```python
from build123d import *

# Parameters (mm, degrees)
F1_DEPTH = 3
F0_W     = 20
F0_H     = 2.5
F0_W_2   = 70
F2_DEPTH = 3
F3_DEPTH = 15
F4_R     = 2


with BuildPart() as f1:
    # F0 (on Top) → F1 (new body)
    with BuildSketch(Plane.XY):
        Polygon((-24.26379, -16.103005), (-24.26379, -22.103005), (-4.26379, -22.103005), (25.73621, -22.103005), (45.73621, -22.103005), (45.73621, -16.103005), align=None)
    extrude(amount=F1_DEPTH)

    # F0 (on Top) → F2 (join)
    with BuildSketch(Plane.XY):
        with Locations((-14.26379, -23.353005)):
            Rectangle(F0_W, F0_H)
        with Locations((35.73621, -23.353005)):
            Rectangle(F0_W, F0_H)
        with Locations((10.73621, -14.853005)):
            Rectangle(F0_W_2, F0_H)
    extrude(amount=F2_DEPTH)

    # F0 (on Top) → F3 (join)
    with BuildSketch(Plane.XY):
        with Locations((10.73621, -14.853005)):
            Rectangle(F0_W_2, F0_H)
        with Locations((-14.26379, -23.353005)):
            Rectangle(F0_W, F0_H)
        with Locations((35.73621, -23.353005)):
            Rectangle(F0_W, F0_H)
    extrude(amount=-F3_DEPTH)

    # F4
    f4_edges = [f1.edges().sort_by_distance(p)[0] for p in [
        (10.73621, -13.603005, 3),
        (-14.26379, -24.603005, 3),
        (35.73621, -24.603005, 3),
    ]]
    fillet(f4_edges, radius=F4_R)


solid = f1.part
```
Geometry: final body of the model. Coordinates: model frame, mm. A direction names the side the tool comes from. Give positions to 0.01 mm unless a question says otherwise; leave off trailing zeros. Loops run counter-clockwise (first coordinate to the right, second up) from the corner with the lowest first, then second, coordinate; pieces in that order, holes last. Notation, with made-up numbers: (28, 81) - (47, 81) arc R15 cw to (47, 96) - close; hole circle Ø11 at (2.25, 52.5). An arc over 180 degrees is marked (long way). Answer as CSV lines item,"result". Start each with the question number.
(1) Reachability of faces 4 (the face through (36, -22.103, -7)), 5 (the face through (10, -19, 3)), 6 (the face through (11, -22.103, 1)) from +Z, -Z, +X, -X, +Y, -Y: full face, straight path, thin tool, end or side. Return the list, or none.
(2) Section query D-D (x = 13). Output: boundary loops of the cut face in (y, z).
(3) Pin query (flat end, axial travel): P1, Ø1.8, axis at x = 5.5, y = -18, coming from the -Z side; P2, Ø7.5, axis at x = 5, z = -6, coming from the -Y side; P3, Ø3.5, axis at x = 14.5, z = 2, coming from the -Y side. Return the tip coordinate at first contact, or that it passes through.
(4) Section query C-C (y = -17.5). Output: boundary loops of the cut face in (x, z), and give its area (3 significant figures).
(5) Mould query, pull axis Y, two halves, no side actions, for faces 1 (the face through (10, -15, -15)), 2 (the face through (10, -13.603, -7)), 3 (the face through (-14, -22.103, -7)). Classes: +Y half, -Y half, draft (parallel to the pull), parting line (faces both ways), or undercut.
(6) Ray query, line 1 along Y through (x, z) = (-19.5, -5.25); line 2 along X through (y, z) = (-24, -2.25); line 3 along Y through (x, z) = (21.5, -13.5). Return the intervals inside material, ascending. Write a range as [from, to].
(7) Section query B-B (x = 40). Output: boundary loops of the cut face in (y, z).
(8) Section query A-A (z = -12.5). Output: boundary loops of the cut face in (x, y).
Worked answers:
1,face 4,"-Z, +X, -X"
1,face 5,"+Z, +X, -X, +Y, -Y"
1,face 6,"+Z, -Z, -Y"
2,outline,"(-22.1, 0) - (-16.1, 0) - (-16.1, -15) - (-13.6, -15) - (-13.6, 1) arc R2 ccw to (-15.6, 3) - (-22.1, 3) - close"
3,P1,"stops at z = 0"
3,P2,"stops at y = -16.1"
3,P3,"stops at y = -22.1"
4,outline,"(-24.26, 0) - (45.74, 0) - (45.74, 3) - (-24.26, 3) - close"
4,area,"210 mm^2"
5,face 1,"draft"
5,face 2,"+Y half"
5,face 3,"undercut"
6,line 1,"y = [-24.6, -22.1], [-16.1, -13.6]"
6,line 2,"x = [-24.26, -4.26], [25.74, 45.74]"
6,line 3,"y = [-16.1, -13.6]"
7,outline,"(-24.6, -15) - (-22.1, -15) - (-22.1, 0) - (-16.1, 0) - (-16.1, -15) - (-13.6, -15) - (-13.6, 1) arc R2 ccw to (-15.6, 3) - (-22.6, 3) arc R2 ccw to (-24.6, 1) - close"
8,outline,"(-24.26, -24.6) - (-4.26, -24.6) - (-4.26, -22.1) - (-24.26, -22.1) - close; (-24.26, -16.1) - (45.74, -16.1) - (45.74, -13.6) - (-24.26, -13.6) - close; (25.74, -24.6) - (45.74, -24.6) - (45.74, -22.1) - (25.74, -22.1) - close"
